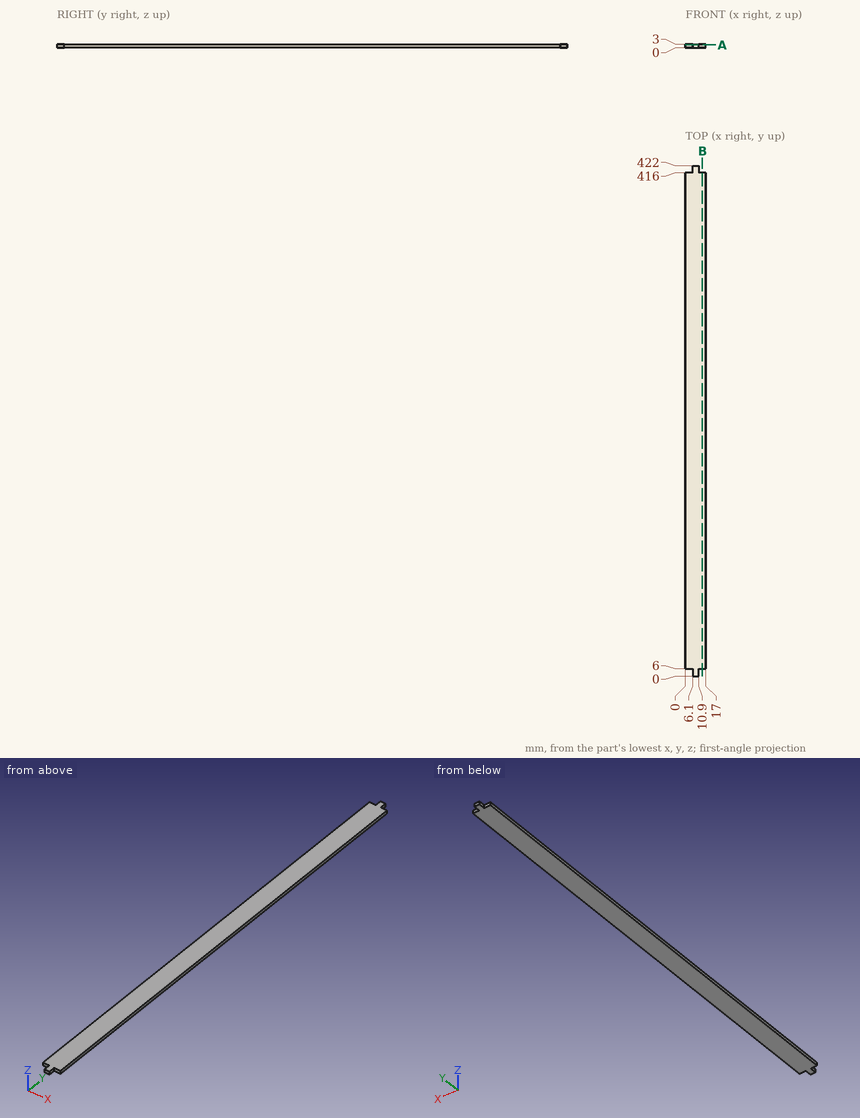
Input: dimensioned drawing with shaded views. Units: mm. Origin: part minimum x, y, z. Give positions to 0.01 mm unless a question says otherwise; leave off trailing zeros. Write each loop counter-clockwise with the first axis right and the second up, starting at its lowest first coordinate (ties: lowest second). Pieces come first, ordered by that corner, then holes.
1. Section query A-A (z = 2.2). Return the cut outline in (x, y), then the cut area to 3 significant figures.
2. Section query B-B (x = 14). Return the cut outline in (y, z), then the cut area to 3 significant figures.
3. First-contact query: pin 1 (0.9 mm diameter, centred on y = 3.5, z = 1, fed in from -X); pin 2 (0.9 mm diameter, centred on x = 1.5, z = 1.5, fed in from +Y); pin 3 (0.9 mm diameter, centred on y = 2, z = 1, fed in from +X). Flat tips, straight axial feed; report the tip coordinate or a pass-through.
4. Material intervals for line 1 along Y through (x, z) = (11, 0.7), sorted ascending.
Output values:
1. outline: (0, 6) - (6.1, 6) - (6.1, 0) - (10.9, 0) - (10.9, 6) - (17, 6) - (17, 416) - (10.9, 416) - (10.9, 422) - (6.1, 422) - (6.1, 416) - (0, 416) - close
1. area: 7,030 mm2
2. outline: (6, 0) - (416, 0) - (416, 3) - (6, 3) - close
2. area: 1,230 mm2
3. pin 1: stops at x = 6.1
3. pin 2: stops at y = 416
3. pin 3: stops at x = 10.9
4. line 1: y = 6 to 416
